The listing builds one solid part. Answer for the finished solid, in the listing's coordinates (mm). Face numbers are marked on the shaded views. Coordinates: 2 decimals unless noted, no trailing zeros. Order: outer loops, then holes, each group sorted by start corner. A loop starts at its lowest first (then second) coordinate and runs counter-clockwise, first axis right, second up. Notation, with made-up numbers: M -6,-23.5 L 0,-23.5 A23 cw 0,-2.5 Z; hole C 86.5,69 d6. An arc over 180 degrees is marked long. One line per item, written item: value. Start each with the question number.
Q1. The part is cut by section B-B on x = 577.5. Give the vertices of the cut face in (y, z), then the cut area to 3 significant figures.
Q2. Determine the mould class of the marked faces 1 and 2 for opening direction X: pulls with the +X half, pulls with the -X half, needs draft (parallel to the pull), parting line crosses it, or undercut.
Q3. Straight lines are drawn through the part: line 1 along X through (y, z) = (15.5, 75); line 2 along Z through (x, y) = (1024.5, 11.75); line 3 along Y through (x, z) = (299.5, 737.5). For each, find the intervals that lie inside material, in ascending order. Write a range as [from, to].
Q4. The part is cut by section A-A on y = 15.5. Give the vertices of the cut face in (x, z).
Q5. The part is cut by section C-C on z = 130.5. Give the vertices of the cut face in (x, y).
Q6. The part is cut by section D-D on z = 879.5. Give the vertices of the cut face in (x, y), then the cut area to 3 significant figures.
Q7. Each of these flat-tipped pins is pushed along its axis until it touches: pin 1 Ø4 at (x, y) = (945.5, 5.5) entering from -Z; pin 2 Ø1.6 at (y, z) = (1, 1093.5) entering from -X; pin 3 Ø1.5 at (x, z) = (981, 357) entering from +Y; pin 4 Ø0.6 at (y, z) = (1.5, 1094.5) entering from +X. Where does it stop, or does it pass through?
```python
from build123d import *

# Parameters (mm, degrees)
BASE_FLANGE1_DEPTH             = 1096
EDGE_FLANGE1_STRIP_W           = 12
EDGE_FLANGE1_STRIP_H           = 2
EDGE_FLANGE1_STRIP_CUT_DEPTH   = 1147
EDGE_FLANGE1_STRIP_2_W         = 12
EDGE_FLANGE1_STRIP_2_H         = 2
EDGE_FLANGE1_STRIP_CUT_2_DEPTH = 1147
EDGE_FLANGE1_DEPTH             = 1147
EDGE_FLANGE1_BEND_DEPTH        = 1147
SKETCH12_R                     = 63.920888045
CUT_EXTRUDE1_DEPTH             = 10


# Sheet-metal steps are written as plain solids
with BuildPart() as part:
    # Sketch1 → Base-Flange1 (new body)
    with BuildSketch(Plane.XY):
        with BuildLine():
            Line((0, 25), (0, 4))
            ThreePointArc((0, 4), (1.171572875, 1.171572875), (4, 0))
            Line((4, 0), (1151, 0))
            ThreePointArc((1151, 0), (1153.828427125, 1.171572875), (1155, 4))
            Line((1155, 4), (1155, 25))
            Line((1155, 25), (1153, 25))
            Line((1153, 25), (1153, 4))
            ThreePointArc((1153, 4), (1152.414213562, 2.585786438), (1151, 2))
            Line((1151, 2), (4, 2))
            ThreePointArc((4, 2), (2.585786438, 2.585786438), (2, 4))
            Line((2, 4), (2, 25))
            Line((2, 25), (0, 25))
        make_face()
    extrude(amount=BASE_FLANGE1_DEPTH)

    # Edge-Flange1 strip (across the edge) → Edge-Flange1 strip cut (cut)
    with BuildSketch(Plane(origin=(4, 2, 1096), x_dir=(0, 0, -1), z_dir=(1, 0, 0))):
        with Locations((-2, -1)):
            Rectangle(EDGE_FLANGE1_STRIP_W, EDGE_FLANGE1_STRIP_H)
    extrude(amount=EDGE_FLANGE1_STRIP_CUT_DEPTH, mode=Mode.SUBTRACT)

    # Edge-Flange1 strip 2 (across the edge) → Edge-Flange1 strip cut 2 (cut)
    with BuildSketch(Plane(origin=(1151, 2, 0), x_dir=(0, 0, 1), z_dir=(-1, 0, 0))):
        with Locations((-2, -1)):
            Rectangle(EDGE_FLANGE1_STRIP_2_W, EDGE_FLANGE1_STRIP_2_H)
    extrude(amount=EDGE_FLANGE1_STRIP_CUT_2_DEPTH, mode=Mode.SUBTRACT)

    # Edge-Flange1 section (across the edge) → Edge-Flange1 (add)
    with BuildSketch(Plane(origin=(4, 2, 1096), x_dir=(0, 0, -1), z_dir=(1, 0, 0))):
        with BuildLine():
            Line((0, 2), (0, 23))
            Line((0, 23), (2, 23))
            Line((2, 23), (2, 2))
            ThreePointArc((2, 2), (2.585786438, 0.585786438), (4, 0))
            Line((4, 0), (4, -2))
            ThreePointArc((4, -2), (1.171572875, -0.828427125), (0, 2))
        make_face()
    extrude(amount=EDGE_FLANGE1_DEPTH)

    # Edge-Flange1 section 2 (across the edge) → Edge-Flange1 bend (add)
    with BuildSketch(Plane(origin=(1151, 2, 0), x_dir=(0, 0, 1), z_dir=(-1, 0, 0))):
        with BuildLine():
            Line((0, 2), (0, 23))
            Line((0, 23), (2, 23))
            Line((2, 23), (2, 2))
            ThreePointArc((2, 2), (2.585786438, 0.585786438), (4, 0))
            Line((4, 0), (4, -2))
            ThreePointArc((4, -2), (1.171572875, -0.828427125), (0, 2))
        make_face()
    extrude(amount=EDGE_FLANGE1_BEND_DEPTH)

    # Sketch12 → Cut-Extrude1 (cut)
    with BuildSketch(Plane(origin=(0, 2, 0), x_dir=(1, 0, 0), z_dir=(0, 1, 0))):
        with Locations(Location((577.5, -840.335133885, 0), (0, 0, 270))):
            Circle(SKETCH12_R)
    extrude(amount=-CUT_EXTRUDE1_DEPTH, mode=Mode.SUBTRACT)


solid = part.part
```
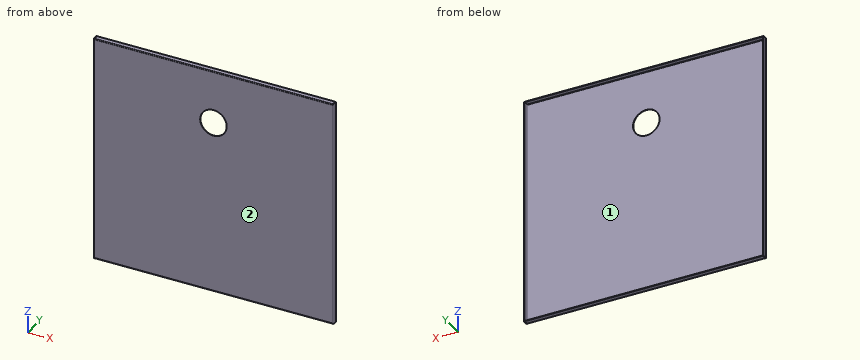
Output:
1. outline: M 0,4 A4 ccw 4,0 L 25,0 L 25,2 L 4,2 A2 cw 2,4 L 2,776.41 L 0,776.41 Z; M 0,904.26 L 2,904.26 L 2,1092 A2 cw 4,1094 L 25,1094 L 25,1096 L 4,1096 A4 ccw 0,1092 Z
1. area: 2,020 mm^2
2. face 1: undercut
2. face 2: needs draft
3. line 1: x = [0, 2], [1153, 1155]
3. line 2: z = [0, 2], [1094, 1096]
3. line 3: y = [0, 2]
4. outline: M 0,0 L 2,0 L 2,1096 L 0,1096 Z; M 4,0 L 1151,0 L 1151,2 L 4,2 Z; M 4,1094 L 1151,1094 L 1151,1096 L 4,1096 Z; M 1153,0 L 1155,0 L 1155,1096 L 1153,1096 Z
5. outline: M 0,4 A4 ccw 4,0 L 1151,0 A4 ccw 1155,4 L 1155,25 L 1153,25 L 1153,4 A2 cw 1151,2 L 4,2 A2 cw 2,4 L 2,25 L 0,25 Z
6. outline: M 0,4 A4 ccw 4,0 L 526.98,0 L 526.98,2 L 4,2 A2 cw 2,4 L 2,25 L 0,25 Z; M 628.02,0 L 1151,0 A4 ccw 1155,4 L 1155,25 L 1153,25 L 1153,4 A2 cw 1151,2 L 628.02,2 Z
6. area: 2,190 mm^2
7. pin 1: stops at z = 0
7. pin 2: stops at x = 0.66
7. pin 3: stops at y = 2
7. pin 4: stops at x = 1154.34
